```python
from build123d import *

# Parameters (mm, degrees)
F2_W     = 101.22
F2_H     = 61.63
F0_W     = 111.14
F0_H     = 75.07
F4_R     = 5
F5_T     = 2.5
F7_DEPTH = 6


# Not quite as in the source:
# - a shell that OpenCascade refuses in one call is made with other operations: the cavity is built on its own and cut out


with BuildPart() as f3:
    # F2 (on offset) → F3 section 0
    with BuildSketch(Plane.XY.offset(42)):
        Rectangle(F2_W, F2_H)
    # F0 (on Top) → F3 section 1
    with BuildSketch(Plane.XY):
        Rectangle(F0_W, F0_H)
    loft()

    # F4
    f4_edges = [f3.edges().sort_by_distance(p)[0] for p in [
        (-53.09, 34.175, 21),
        (53.09, 34.175, 21),
        (53.09, -34.175, 21),
        (-53.09, -34.175, 21),
        (0, -30.815, 42),
        (50.61, 0, 42),
        (0, 30.815, 42),
        (-50.61, 0, 42),
    ]]
    fillet(f4_edges, radius=F4_R)

    # F5: shell of thickness 2.5, made by hand


with BuildPart() as f5_core1:
    # F5_t2: copy of F3
    add(f3.part)

    # the walls: a layer under each face that stays
    f5_faces = [f5_core1.faces().sort_by_distance(p)[0] for p in [
        (-53.3506124987, 0, 18.7932006155),
        (-51.8873286605, 33.0489229278, 18.9750242391),
        (-51.8873286605, -33.0489229278, 18.9750242391),
        (-49.4874767675, 0, 40.7371115956),
        (0, 34.5118037996, 18.8949762528),
        (0, -34.5118037996, 18.8949762528),
        (51.8873286605, 33.0489229278, 18.9750242391),
        (51.8873299173, -33.0489246306, 18.9750135967),
        (53.3506124987, 0, 18.7932006155),
        (-48.5145599261, 28.9002335794, 40.7371115784),
        (-48.5145599261, -28.9002335794, 40.7371115784),
        (0, 0, 42),
        (0, 29.7956483786, 40.8045868716),
        (0, -29.7956483786, 40.8045868716),
        (48.5145600153, 28.9002373676, 40.7371091413),
        (48.5145599261, -28.9002335794, 40.7371115784),
        (49.4874767675, 0, 40.7371115956),
    ]]
    thicken(f5_faces, amount=-F5_T, mode=Mode.SUBTRACT)


with BuildPart() as f3_1:
    add(f3.part)

    # what is left inside the walls is the cavity
    f5_cavity = [f5_core1.part.solids().sort_by_distance(p)[0] for p in [
        (10.775811, 15.952675, 0.025),
    ]]
    add(f5_cavity, mode=Mode.SUBTRACT)

    # F6 (on face) → F7 (join)
    with BuildSketch(Plane(origin=(0, 0, 0), x_dir=(1, 0, 0), z_dir=(0, 0, -1))):
        with BuildLine():
            Line((52.57, 39.535), (-52.57, 39.535))
            ThreePointArc((-52.57, 39.535), (-56.1055339059, 38.0705339059), (-57.57, 34.535))
            Line((-57.57, 34.535), (-57.57, -34.535))
            ThreePointArc((-57.57, -34.535), (-56.1055339059, -38.0705339059), (-52.57, -39.535))
            Line((-52.57, -39.535), (52.57, -39.535))
            ThreePointArc((52.57, -39.535), (56.1055339059, -38.0705339059), (57.57, -34.535))
            Line((57.57, -34.535), (57.57, 34.535))
            ThreePointArc((57.57, 34.535), (56.1055339059, 38.0705339059), (52.57, 39.535))
        make_face()
    extrude(amount=F7_DEPTH)


solid = f3_1.part
```
For this review, take the finished solid that the model builds, in its own axes (mm). A direction names the side the tool comes from. Give positions to 0.01 mm unless a question says otherwise; leave off trailing zeros. Answer as a JSON object with one key per item and string values. Group by question number.
Item 1: For pin 1 Ø12 at (x, z) = (-9, 36.5) entering from +Y (3 decimals); pin 2 Ø3 at (x, z) = (8, 14.5) entering from +Y (3 decimals); pin 3 Ø1.5 at (x, z) = (16.5, 21.5) entering from +Y (3 decimals), all flat-tipped, find the tip position at first contact; note any pin that passes through.
Item 2: For probe 1 along Z at (x, y) = (15, -14.5); probe 2 along X at (y, z) = (0, 18); probe 3 along X at (y, z) = (-28, 13), list the stretches that pass through material, from the lowest coordinate up. Write a range as [from, to].
Item 3: Tool access review of faces 1 (the flat face through (-1, 0, 39.5)), 2 (the flat face through (57.57, 0, -3)): name each direction out of +Z, -Z, +X, -X, +Y, -Y from which nothing blocks a thin tool from reaching the whole face with its end or side.
Item 4: Draft analysis for pull direction X (two halves, no side actions). For faces 3 (the flat face through (-50.88, 0.46, 18.39)), 4 (the flat face through (-1, 0, 42)), 5 (the cylindrical face through (-56.066, -38.109, -2.958)), state which applies: +X half, -X half, draft (parallel to the pull), parting line (faces both ways), or undercut.
Check result:
{
 "1": {"pin 1": "stops at y = 32.655", "pin 2": "stops at y = 35.455", "pin 3": "stops at y = 34.215"},
 "2": {"probe 1": "z = [-6, 0], [39.5, 42]", "probe 2": "x = [-53.44, -50.93], [50.93, 53.44]", "probe 3": "x = [-54.03, -51.52], [51.52, 54.03]"},
 "3": {"face 1": "none", "face 2": "+Z, -Z, +X, +Y, -Y"},
 "4": {"face 3": "undercut", "face 4": "draft", "face 5": "-X half"}
}
